Here's how the part is built. I have some questions about the finished solid (model axes, mm). Give positions to 0.01 mm unless a question says otherwise; leave off trailing zeros. Loops run counter-clockwise (first coordinate to the right, second up) from the corner with the lowest first, then second, coordinate; pieces in that order, holes last.
Q1. If we section it at A-A (z = 22): Please give me the cut outline in (x, y), plus the area to 3 significant figures.
Q2. If we section it at B-B (y = 28.5): Please give me the cut outline in (x, z).
Q3. I need wall thicknesses on line 1 (X direction, y = 49.5, z = 12.25); line 2 (Y direction, x = 100.5, z = 10); line 3 (X direction, y = 133.5, z = 10.25). Which ranges of each line are inside material? Lowest first, please.
Q4. Will these pins go through, and if not, where does the flat tip stop? P1, Ø6, axis at y = 84.5, z = 4, coming from the +X side; P2, Ø1.5, axis at y = 111, z = 5, coming from the -X side; P3, Ø6, axis at x = 104.5, z = 19, coming from the -Y side; P4, Ø12, axis at x = 79, y = 48.5, coming from the +Z side.
from build123d import *

# Parameters (mm, degrees)
F2_DEPTH = 25.4
F3_R     = 25.39999


# Not quite as in the source:
# - a fillet or chamfer is up to 0.001 mm smaller than in the source, because OpenCascade refuses the exact size


with BuildPart() as f2:
    # F1 (on face) → F2 (new body)
    with BuildSketch(Plane.XY):
        with BuildLine():
            Line((180.582366013, 140.1712134682), (40.4111525448, 0))
            Line((40.4111525448, 0), (80.8223050896, 0))
            Line((80.8223050896, 0), (196.9228733519, 116.1005682623))
            ThreePointArc((196.9228733519, 116.1005682623), (189.1359310844, 128.3961041965), (180.582366013, 140.1712134682))
        make_face()
    extrude(amount=F2_DEPTH)

    # F3 (radius 25.4 in the source; OpenCascade refuses exactly that, so slightly less here)
    f3_edges = [f2.edges().sort_by_distance(p)[0] for p in [
        (189.135931, 128.396104, 25.4),
    ]]
    fillet(f3_edges, radius=F3_R)


solid = f2.part
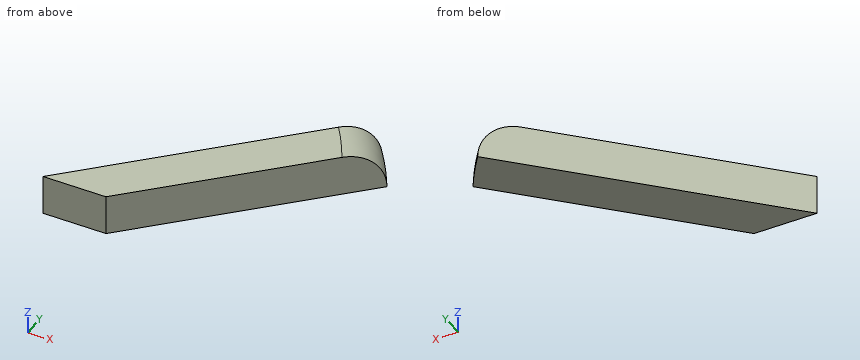
Check sheet entries:
1. outline: (40.41, 0) - (80.82, 0) - (187.63, 106.8) arc R215.89 ccw to (171.52, 131.11) - close
1. area: 4,820 mm2
2. outline: (68.91, 0) - (109.32, 0) - (109.32, 25.4) - (68.91, 25.4) - close
3. line 1: x = 89.91 to 130.32
3. line 2: y = 19.68 to 60.09
3. line 3: x = 173.91 to 182.9
4. P1: stops at x = 168.32
4. P2: stops at x = 150.66
4. P3: stops at y = 20.68
4. P4: passes through
